The figure shows three views and two pictorial views of one solid part (mm, origin at its lowest corner). Answer the questions. A direction names the side the tool comes from. Coordinates: 2 decimals unless noted, no trailing zeros. Write each loop counter-clockwise with the first axis right and the second up, starting at its lowest first coordinate (ties: lowest second). Pieces come first, ordered by that corner, then holes.
Item 1: Section A-A (z = 1) is taken. Give the vertices of the cut face in (x, y).
Item 2: Determine the mould class of the marked faces 1, 2 and 3 for opening direction Y: released by +Y, released by -Y, zero draft, split by the parting line, or undercut.
Item 3: Straight lines are drawn through the part: probe 1 along Y at (x, z) = (4, 5.3); probe 2 along X at (y, z) = (4, 5); probe 3 along Z at (x, y) = (6, 20.5). For each, find the intervals that lie inside material, in ascending order.
Item 4: Section D-D (y = 13) is taken. Give the vertices of the cut face in (x, z).
Item 5: A tool of negligible diameter and unlimited length cuts with its end or side. For the marked faces 4, 5 and 6, from which of +Z, -Z, +X, -X, +Y, -Y can it reach the whole face along a straight path? Write none if from no direction.
Item 6: Section B-B (x = 3.5) is taken. Give the vertices of the cut face in (y, z) (1 decimal).
Item 7: Section C-C (z = 5.5) is taken. Give the vertices of the cut face in (x, y).
Item 8: Each of these flat-tipped pins is pushed along its axis until it touches: P1, Ø2, axis at x = 2.5, y = 15.5, coming from the -Z side; P2, Ø3, axis at x = 4, y = 4, coming from the +Z side. Where does it stop, or does it pass through?
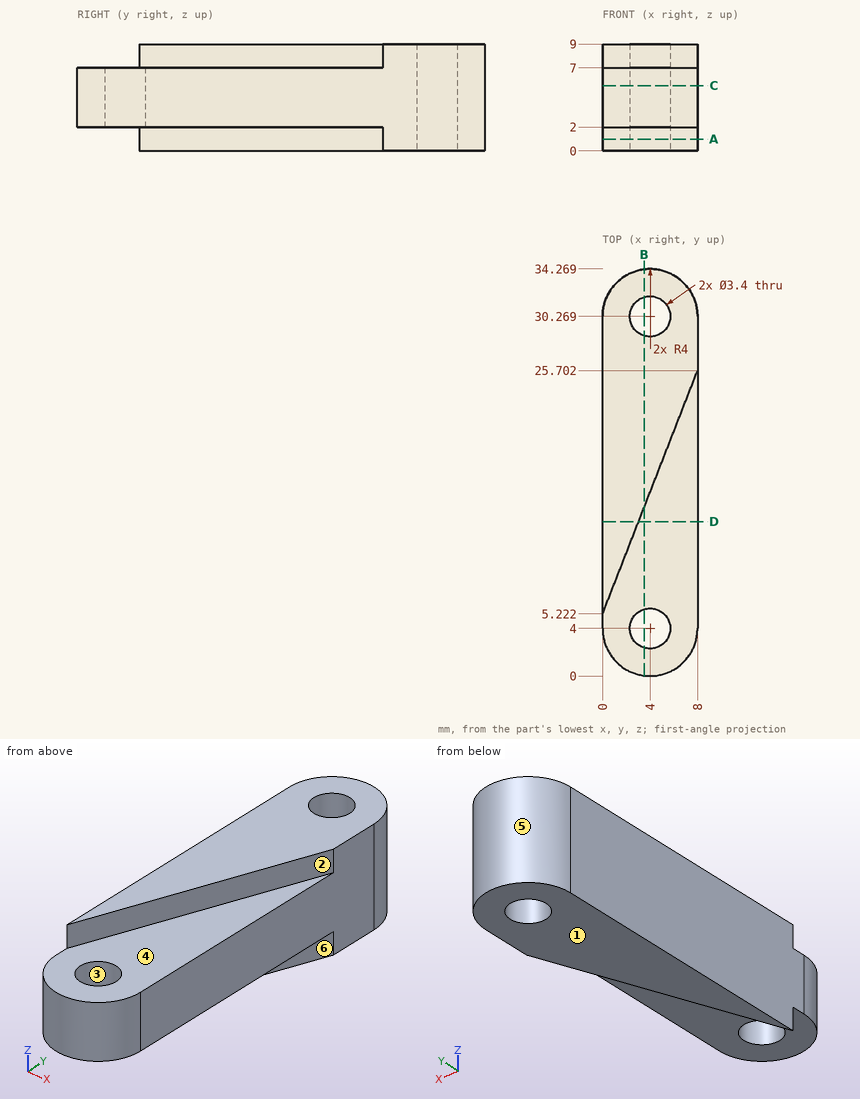
Established:
1. outline: (0, 5.22) - (8, 25.7) - (8, 30.27) arc R4 ccw to (0, 30.27) - close; hole circle Ø3.4 at (4, 30.27)
2. face 1: zero draft
2. face 2: released by -Y
2. face 3: undercut
3. probe 1: y = 0 to 2.3, 5.7 to 28.57, 31.97 to 34.27
3. probe 2: x = 0 to 2.3, 5.7 to 8
3. probe 3: z = 2 to 7
4. outline: (0, 0) - (3.04, 0) - (3.04, 2) - (8, 2) - (8, 7) - (3.04, 7) - (3.04, 9) - (0, 9) - close
5. face 4: +Z, +X, -Y
5. face 5: +Z, -Z, +Y
5. face 6: -Z, +X, -Y
6. outline: (0, 2) - (2.4, 2) - (2.4, 7) - (0, 7) - close; (5.6, 2) - (14.2, 2) - (14.2, 0) - (28.6, 0) - (28.6, 9) - (14.2, 9) - (14.2, 7) - (5.6, 7) - close; (31.9, 0) - (34.2, 0) - (34.2, 9) - (31.9, 9) - close
7. outline: (0, 4) arc R4 ccw to (8, 4) - (8, 30.27) arc R4 ccw to (0, 30.27) - close; hole circle Ø3.4 at (4, 4); hole circle Ø3.4 at (4, 30.27)
8. P1: stops at z = 0
8. P2: passes through
